Input: part model. Units: mm. Frame: model coordinates. A direction names the side the tool comes from. Round coordinates to 2 decimals unless told otherwise and drop trailing zeros. Loops run counter-clockwise (first coordinate to the right, second up) from the corner with the lowest first, then second, coordinate; pieces in that order, holes last. Notation, with made-up numbers: (46, 36) -> (101, 36) arc R21 cw to (101, 64) -> close; hole circle Ø5 at (31, -22). An arc over 180 degrees is marked (long way). Answer in a Markdown table with one row per item. Add a question column.
Q1. Pin query (flat end, axial travel): pin 1 (7 mm diameter, centred on x = 71.92, y = 12, fed in from -Z); pin 2 (3 mm diameter, centred on x = 49.5, y = -25, fed in from -Z). Return the tip coordinate at first contact, or that it passes through.
Q2. Ray query, L1, parallel to X at y = -4.5, z = -0.8; L2, parallel to X at y = 11.5, z = -0.9; L3, parallel to X at y = 14, z = -0.9. Return the intervals inside material, ascending. Write a range as from..to.
Q3. Section B-B, the plane y = -0.5. Output: boundary loops of the cut face in (x, z).
Q4. Section C-C, the plane x = 9.5. Output: boundary loops of the cut face in (y, z), and give its area (3 significant figures).
Q5. Reachability of faces 1 (the face through (-74.85, 35.98, -2.61)), 2 (the face through (-75.033, 18.934, -0.74)) from +Z, -Z, +X, -X, +Y, -Y: full face, straight path, thin tool, end or side. Return the list, or none.
Q6. Mould query, pull axis X, two halves, no side actions, for faces 3 (the face through (76, -36.07, -1.12)), 4 (the face through (-71, 37, -3.75)), 5 (the face through (74.54, 12.83, -0.74)). Classes: pulls with the +X half, pulls with the -X half, needs draft (parallel to the pull), parting line crosses it, or undercut.
Q7. Section D-D, the plane y = 12. Output: boundary loops of the cut face in (x, z).
```python
from build123d import *

# Parameters (mm, degrees)
F0_R     = 0.5
F0_R_2   = 9.875
F0_W     = 105.670338
F0_H     = 70.447
F0_R_3   = 2.75
F0_R_4   = 2
F0_R_5   = 1
F1_DEPTH = 1.5
F2_R     = 0.75
F3_R     = 0.5
F4_R     = 0.5
F6_DEPTH = 2.25


with BuildPart() as f1:
    # F0 (on Top) → F1 (new body)
    with BuildSketch(Plane.XY):
        with BuildLine():
            ThreePointArc((77.5, 32.5), (76.035534, 36.035534), (72.5, 37.5))
            Line((72.5, 37.5), (-72.5, 37.5))
            ThreePointArc((-72.5, 37.5), (-76.035534, 36.035534), (-77.5, 32.5))
            Line((-77.5, 32.5), (-77.5, -32.5))
            ThreePointArc((-77.5, -32.5), (-76.035534, -36.035534), (-72.5, -37.5))
            Line((-72.5, -37.5), (72.5, -37.5))
            ThreePointArc((72.5, -37.5), (76.035534, -36.035534), (77.5, -32.5))
            Line((77.5, -32.5), (77.5, 32.5))
        make_face()
        with Locations((-69.937184, -32)):
            Circle(F0_R, mode=Mode.SUBTRACT)
        with Locations((-72.5, -29.437184)):
            Circle(F0_R, mode=Mode.SUBTRACT)
        with Locations((-68.125, -30.3125)):
            Circle(F0_R, mode=Mode.SUBTRACT)
        with Locations((-66.312816, -32)):
            Circle(F0_R, mode=Mode.SUBTRACT)
        with Locations((-63.75, -29.437184)):
            Circle(F0_R, mode=Mode.SUBTRACT)
        with Locations((-70.8125, -27.625)):
            Circle(F0_R, mode=Mode.SUBTRACT)
        with Locations((-68.125, -27.625)):
            Circle(F0_R, mode=Mode.SUBTRACT)
        with Locations((-72.5, -25.812816)):
            Circle(F0_R, mode=Mode.SUBTRACT)
        with Locations((-68.125, -24.9375)):
            Circle(F0_R, mode=Mode.SUBTRACT)
        with Locations((-65.4375, -27.625)):
            Circle(F0_R, mode=Mode.SUBTRACT)
        with Locations((-63.75, -25.812816)):
            Circle(F0_R, mode=Mode.SUBTRACT)
        with Locations((-69.937184, -23.25)):
            Circle(F0_R, mode=Mode.SUBTRACT)
        with Locations((-66.312816, -23.25)):
            Circle(F0_R, mode=Mode.SUBTRACT)
        Polygon((-68.167584, -4), (-68.167584, 2), (-62.667584, 2), (-62.667584, -4), (-56.667584, -4), (-56.667584, -9.5), (-62.667584, -9.5), (-62.667584, -15.5), (-68.167584, -15.5), (-68.167584, -9.5), (-74.167584, -9.5), (-74.167584, -4), align=None, mode=Mode.SUBTRACT)
        with Locations((66.312816, -32)):
            Circle(F0_R, mode=Mode.SUBTRACT)
        with Locations((63.75, -29.437184)):
            Circle(F0_R, mode=Mode.SUBTRACT)
        with Locations((69.937184, -32)):
            Circle(F0_R, mode=Mode.SUBTRACT)
        with Locations((68.125, -30.3125)):
            Circle(F0_R, mode=Mode.SUBTRACT)
        with Locations((72.5, -29.437184)):
            Circle(F0_R, mode=Mode.SUBTRACT)
        with Locations((65.4375, -27.625)):
            Circle(F0_R, mode=Mode.SUBTRACT)
        with Locations((63.75, -25.812816)):
            Circle(F0_R, mode=Mode.SUBTRACT)
        with Locations((68.125, -27.625)):
            Circle(F0_R, mode=Mode.SUBTRACT)
        with Locations((70.8125, -27.625)):
            Circle(F0_R, mode=Mode.SUBTRACT)
        with Locations((72.5, -25.812816)):
            Circle(F0_R, mode=Mode.SUBTRACT)
        with Locations((68.125, -24.9375)):
            Circle(F0_R, mode=Mode.SUBTRACT)
        with Locations((66.312816, -23.25)):
            Circle(F0_R, mode=Mode.SUBTRACT)
        with Locations((69.937184, -23.25)):
            Circle(F0_R, mode=Mode.SUBTRACT)
        with Locations((-65.167584, 18.5)):
            Circle(F0_R_2, mode=Mode.SUBTRACT)
        Rectangle(F0_W, F0_H, mode=Mode.SUBTRACT)
        with Locations((65.1675, 5.25)):
            Circle(F0_R_3, mode=Mode.SUBTRACT)
        with Locations((58.4175, 12)):
            Circle(F0_R_3, mode=Mode.SUBTRACT)
        with Locations((71.9175, 12)):
            Circle(F0_R_3, mode=Mode.SUBTRACT)
        with Locations((65.1675, 18.75)):
            Circle(F0_R_3, mode=Mode.SUBTRACT)
        with Locations((57.835169, 30)):
            Circle(F0_R_4, mode=Mode.SUBTRACT)
        with Locations((55.835169, 34.5)):
            Circle(F0_R_5, mode=Mode.SUBTRACT)
        with Locations((59.835169, 34.5)):
            Circle(F0_R_5, mode=Mode.SUBTRACT)
    extrude(amount=-F1_DEPTH)

    # F2
    f2_edges = [f1.edges().sort_by_distance(p)[0] for p in [
        (0, -37.5, 0),
    ]]
    fillet(f2_edges, radius=F2_R)

    # F3
    f3_edges = [f1.edges().sort_by_distance(p)[0] for p in [
        (-52.835169, 35.2235, -0.75),
        (52.835169, 35.2235, -0.75),
        (-52.835169, -35.2235, -0.75),
        (52.835169, -35.2235, -0.75),
    ]]
    fillet(f3_edges, radius=F3_R)

    # F4
    f4_edges = [f1.edges().sort_by_distance(p)[0] for p in [
        (-68.167584, 2, -0.75),
        (-68.167584, -4, -0.75),
        (-74.167584, -4, -0.75),
        (-62.667584, -4, -0.75),
        (-68.167584, -9.5, -0.75),
        (-62.667584, -15.5, -0.75),
        (-62.667584, -9.5, -0.75),
        (-56.667584, -9.5, -0.75),
        (-56.667584, -4, -0.75),
        (-62.667584, 2, -0.75),
        (-74.167584, -9.5, -0.75),
        (-68.167584, -15.5, -0.75),
    ]]
    fillet(f4_edges, radius=F4_R)

    # F5 (on face) → F6 (join)
    with BuildSketch(Plane(origin=(0, 0, -1.5), x_dir=(1, 0, 0), z_dir=(0, 0, -1))):
        with BuildLine():
            Line((-63.75, -37.5), (-63.55, -37.5))
            ThreePointArc((-63.55, -37.5), (-63.691421, -37.441421), (-63.75, -37.3))
            Line((-63.75, -37.3), (-63.75, -36.9))
            ThreePointArc((-63.75, -36.9), (-63.691421, -36.758579), (-63.55, -36.7))
            Line((-63.55, -36.7), (-63.75, -36.7))
            Line((-63.75, -36.7), (-72.5, -36.7))
            ThreePointArc((-72.5, -36.7), (-74.877051, -35.962604), (-76.419423, -34.009346))
            ThreePointArc((-76.419423, -34.009346), (-76.415534, -34.14204), (-76.495587, -34.247938))
            Line((-76.495587, -34.247938), (-76.836386, -34.473767))
            ThreePointArc((-76.836386, -34.473767), (-77.005927, -34.498128), (-77.132147, -34.382342))
            ThreePointArc((-77.132147, -34.382342), (-75.291799, -36.647994), (-72.5, -37.5))
            Line((-72.5, -37.5), (-63.75, -37.5))
        make_face()
        with BuildLine():
            Line((63.75, -37.5), (72.5, -37.5))
            Line((72.5, -37.5), (72.5, -36.7))
            Line((72.5, -36.7), (63.75, -36.7))
            Line((63.75, -36.7), (63.55, -36.7))
            ThreePointArc((63.55, -36.7), (63.691421, -36.758579), (63.75, -36.9))
            Line((63.75, -36.9), (63.75, -37.3))
            ThreePointArc((63.75, -37.3), (63.691421, -37.441421), (63.55, -37.5))
            Line((63.55, -37.5), (63.75, -37.5))
        make_face()
        with BuildLine():
            Line((72.5, -36.7), (72.5, -37.5))
            ThreePointArc((72.5, -37.5), (74.672226, -37.003491), (76.413041, -35.612573))
            Line((76.413041, -35.612573), (75.786954, -35.114561))
            ThreePointArc((75.786954, -35.114561), (74.32467, -36.282933), (72.5, -36.7))
        make_face()
        with BuildLine():
            Line((75.786954, -35.114561), (76.413041, -35.612573))
            ThreePointArc((76.413041, -35.612573), (76.497426, -35.318286), (76.349003, -35.050524))
            Line((76.349003, -35.050524), (76.291232, -35.012242))
            ThreePointArc((76.291232, -35.012242), (76.020457, -34.971555), (75.786954, -35.114561))
        make_face()
        with BuildLine():
            ThreePointArc((76.349003, -35.050524), (76.497426, -35.318286), (76.413041, -35.612573))
            ThreePointArc((76.413041, -35.612573), (76.544309, -35.439994), (76.667971, -35.261887))
            Line((76.667971, -35.261887), (76.349003, -35.050524))
        make_face()
        with BuildLine():
            ThreePointArc((76.291232, -35.012242), (76.320948, -35.03013), (76.349003, -35.050524))
            Line((76.349003, -35.050524), (76.667971, -35.261887))
            ThreePointArc((76.667971, -35.261887), (76.921981, -34.833684), (77.132147, -34.382342))
            ThreePointArc((77.132147, -34.382342), (77.005927, -34.498128), (76.836386, -34.473767))
            Line((76.836386, -34.473767), (76.495587, -34.247938))
            ThreePointArc((76.495587, -34.247938), (76.415534, -34.14204), (76.419423, -34.009346))
            ThreePointArc((76.419423, -34.009346), (76.232333, -34.426056), (76.001096, -34.819985))
            Line((76.001096, -34.819985), (76.291232, -35.012242))
        make_face()
        with BuildLine():
            ThreePointArc((76.001096, -34.819985), (75.897219, -34.969595), (75.786954, -35.114561))
            ThreePointArc((75.786954, -35.114561), (76.020457, -34.971555), (76.291232, -35.012242))
            Line((76.291232, -35.012242), (76.001096, -34.819985))
        make_face()
    extrude(amount=F6_DEPTH)


solid = f1.part
```
Answer block:
| question | item | result |
|---|---|---|
| 1 | pin 1 | z = -1.5 |
| 1 | pin 2 | through |
| 2 | L1 | -77.5..-74.17, -56.67..-52.84, 52.84..77.5 |
| 2 | L2 | -77.5..-72.13, -58.2..-52.84, 52.84..55.71, 61.12..69.21, 74.62..77.5 |
| 2 | L3 | -77.5..-73.96, -56.38..-52.84, 52.84..56.53, 60.3..70.03, 73.8..77.5 |
| 3 | outline | (-77.5, -1.5) -> (-68.17, -1.5) -> (-68.17, 0) -> (-76.75, 0) arc R0.75 ccw to (-77.5, -0.75) -> close; (-62.67, -1.5) -> (-52.84, -1.5) -> (-52.84, 0) -> (-62.67, 0) -> close; (52.84, -1.5) -> (77.5, -1.5) -> (77.5, -0.75) arc R0.75 ccw to (76.75, 0) -> (52.84, 0) -> close |
| 4 | outline | (-37.5, -1.5) -> (-35.22, -1.5) -> (-35.22, 0) -> (-36.75, 0) arc R0.75 ccw to (-37.5, -0.75) -> close; (35.22, -1.5) -> (37.5, -1.5) -> (37.5, -0.75) arc R0.75 ccw to (36.75, 0) -> (35.22, 0) -> close |
| 4 | area | 6.59 mm^2 |
| 5 | face 1 | -Z, -Y |
| 5 | face 2 | +Z, -Z |
| 6 | face 3 | pulls with the +X half |
| 6 | face 4 | needs draft |
| 6 | face 5 | undercut |
| 7 | outline | (-77.5, -1.5) -> (-72.6, -1.5) -> (-72.6, 0) -> (-76.75, 0) arc R0.75 ccw to (-77.5, -0.75) -> close; (-57.73, -1.5) -> (-52.84, -1.5) -> (-52.84, 0) -> (-57.73, 0) -> close; (52.84, -1.5) -> (55.67, -1.5) -> (55.67, 0) -> (52.84, 0) -> close; (61.17, -1.5) -> (69.17, -1.5) -> (69.17, 0) -> (61.17, 0) -> close; (74.67, -1.5) -> (77.5, -1.5) -> (77.5, -0.75) arc R0.75 ccw to (76.75, 0) -> (74.67, 0) -> close |
